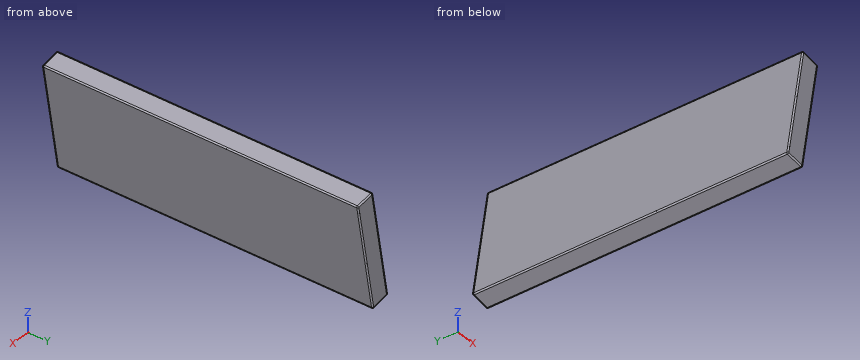
```python
from build123d import *

# Parameters (mm, degrees)
F1_DEPTH = 650
F2_R     = 5


with BuildPart() as f1:
    # F0 (on Front) → F1 (new body, symmetric)
    with BuildSketch(Plane.XZ):
        Polygon((-40, -225), (40, 225), (-38.765001, 239.002667), (-118.765001, -210.997333), align=None)
    extrude(amount=F1_DEPTH, both=True)

    # F2
    f2_edges = [f1.edges().sort_by_distance(p)[0] for p in [
        (40, 0, 225),
        (-38.765001, 0, 239.002667),
        (0.6175, -650, 232.001333),
        (0, -650, 0),
        (-78.765001, -650, 14.002667),
        (-79.3825, -650, -217.998667),
        (-40, 0, -225),
        (-118.765001, 0, -210.997333),
        (-79.3825, 650, -217.998667),
        (0, 650, 0),
        (0.6175, 650, 232.001333),
        (-78.765001, 650, 14.002667),
    ]]
    fillet(f2_edges, radius=F2_R)


solid = f1.part
```
Part model, mm, in its own coordinate system. Round coordinates to 2 decimals unless told otherwise and drop trailing zeros. Order: outer loops, then holes, each group sorted by start corner. A loop starts at its lowest first (then second) coordinate and runs counter-clockwise, first axis right, second up. Notation, with made-up numbers: M 75.5,6.5 L 126.5,6.5 A30 ccw 126.5,29.5 Z; hole C 50,-7 d7. An arc over 180 degrees is marked long. Answer in a Markdown table with one row per item. Add a question column.
Q1. Wall check: L1, parallel to X at y = -228, z = 165.5; L2, parallel to X at y = 200.5, z = 84. Give the ranges that are in metal, low to high. Write a range as from..to.
Q2. Pin check, flat tips, straight feed: pin 1 (10 mm diameter, centred on x = 5.5, y = 263.5, fed in from +Z); pin 2 (1.5 mm diameter, centred on y = 392.5, z = -80, fed in from +X); pin 3 (3 mm diameter, centred on y = 234, z = -69, fed in from +X). Stop position of each tip, or through.
Q3. Cut at A-A on y = -562.5. Give the cut face in (x, z), and give its area (3 significant figures).
Established:
| question | item | result |
|---|---|---|
| 1 | L1 | x = -51.83..29.42 |
| 1 | L2 | x = -66.32..14.93 |
| 2 | pin 1 | stops at z = 232.02 |
| 2 | pin 2 | stops at x = -14.09 |
| 2 | pin 3 | stops at x = -12 |
| 3 | outline | M -117.89,-206.07 A5 ccw -113.84,-211.87 L -44.92,-224.12 A5 ccw -39.12,-220.08 L 39.12,220.08 A5 ccw 35.08,225.88 L -33.84,238.13 A5 ccw -39.64,234.08 Z |
| 3 | area | 36,500 mm2 |
